from build123d import *

# Parameters (mm, degrees)
SKETCH1_W               = 24.5
SKETCH1_H               = 34.22
BOSS_EXTRUDE1_DEPTH     = 7.5
SKETCH2_W               = 24.5
SKETCH2_H               = 34.22
CUT_EXTRUDE1_DEPTH      = 2.86
SKETCH3_W               = 13.25
SKETCH3_H               = 14.15
CUT_EXTRUDE2_DEPTH      = 3.2
BOSS_EXTRUDE2_START     = -18.25
BOSS_EXTRUDE2_DEPTH     = 36.5
BOSS_EXTRUDE2_START_2   = 7.5
BOSS_EXTRUDE2_2_DEPTH   = 4.5
CUT_EXTRUDE3_DEPTH      = 28.465218004
CUT_EXTRUDE3_DEPTH_BACK = 28.465218004
SKETCH4_R               = 7.25
FILLET1_R               = 6
SKETCH6_R               = 1.475
CUT_EXTRUDE4_DEPTH      = 3


with BuildPart() as part:
    # Sketch1 → Boss-Extrude1 (new body)
    with BuildSketch(Plane.XY):
        Polygon((-12.25, -17.11), (-12.25, 17.11), (12.25, 17.11), (12.25, -17.11), (18.25, -17.11), (14.75, 19.61), (-14.75, 19.61), (-18.25, -17.11), align=None)
        Rectangle(SKETCH1_W, SKETCH1_H)
    extrude(amount=BOSS_EXTRUDE1_DEPTH)

    # Sketch2 → Cut-Extrude1 (cut)
    with BuildSketch(Plane(origin=(0, 0, 0), x_dir=(-1, 0, 0), z_dir=(0, 0, -1))):
        Rectangle(SKETCH2_W, SKETCH2_H)
    extrude(amount=-CUT_EXTRUDE1_DEPTH, mode=Mode.SUBTRACT)

    # Sketch3 → Cut-Extrude2 (cut)
    with BuildSketch(Plane(origin=(0, 0, 2.86), x_dir=(-1, 0, 0), z_dir=(0, 0, -1))):
        with BuildLine():
            Line((-6.625, 6.22), (-6.625, 10.62))
            Line((-6.625, 10.62), (-9.525, 10.62))
            ThreePointArc((-9.525, 10.62), (-11.725, 8.42), (-9.525, 6.22))
            Line((-9.525, 6.22), (-6.625, 6.22))
        make_face()
        with Locations((0, 8.42)):
            Rectangle(SKETCH3_W, SKETCH3_H)
        with BuildLine():
            Line((9.525, 10.62), (6.625, 10.62))
            Line((6.625, 10.62), (6.625, 6.22))
            Line((6.625, 6.22), (9.525, 6.22))
            ThreePointArc((9.525, 6.22), (11.725, 8.42), (9.525, 10.62))
        make_face()
    extrude(amount=-CUT_EXTRUDE2_DEPTH, mode=Mode.SUBTRACT)

    # Boss-Extrude2: read off the stored shape, not the designer's step
    # Boss-Extrude2 outline → Boss-Extrude2 (add)
    with BuildSketch(Plane.YZ.offset(BOSS_EXTRUDE2_START)):
        Polygon((-17.11, 11.359427519), (-17.11, 7.5), (19.61, 7.5), align=None)
    extrude(amount=BOSS_EXTRUDE2_DEPTH)

    # Boss-Extrude2 2 outline → Boss-Extrude2 2 (cut)
    with BuildSketch(Plane.XY.offset(BOSS_EXTRUDE2_START_2)):
        Polygon((14.75, 19.61), (18.25, -17.11), (18.25, 21), (14.617510893, 21), align=None)
        Polygon((-14.75, 19.61), (-14.617510893, 21), (-18.25, 21), (-18.25, -17.11), align=None)
    extrude(amount=BOSS_EXTRUDE2_2_DEPTH, mode=Mode.SUBTRACT)

    # Sketch4 → Cut-Extrude3 (cut, two sides: drawn at the far end of the back side and taken through both)
    with BuildSketch(Plane(origin=(0, 0, 6.06), x_dir=(-1, 0, 0), z_dir=(0, 0, -1)).offset(-CUT_EXTRUDE3_DEPTH_BACK)):
        with Locations(Location((0, 8.42, 0), (0, 0, 17.6648328))):
            Circle(SKETCH4_R)
    extrude(amount=CUT_EXTRUDE3_DEPTH + CUT_EXTRUDE3_DEPTH_BACK, mode=Mode.SUBTRACT)

    # Fillet1
    fillet1_edges = [part.edges().sort_by_distance(p)[0] for p in [
        (-14.75, 19.61, 3.75),
        (14.75, 19.61, 3.75),
    ]]
    fillet(fillet1_edges, radius=FILLET1_R)

    # Sketch6 → Cut-Extrude4 (cut)
    with BuildSketch(Plane(origin=(0, 0, 2.86), x_dir=(-1, 0, 0), z_dir=(0, 0, -1))):
        with Locations((-10.2, 14.86)):
            Circle(SKETCH6_R)
        with Locations(Location((10.2, 14.86, 0), (0, 0, 180))):
            Circle(SKETCH6_R)
    extrude(amount=-CUT_EXTRUDE4_DEPTH, mode=Mode.SUBTRACT)


solid = part.part
Read the model definition and answer for the solid it produces. Units are mm, in the model's axes. A direction names the side the tool comes from. Give positions to 0.01 mm unless a question says otherwise; leave off trailing zeros. Loops run counter-clockwise (first coordinate to the right, second up) from the corner with the lowest first, then second, coordinate; pieces in that order, holes last. Notation, with made-up numbers: M 52.5,19 L 57.5,19 A14 ccw 57.5,27 Z; hole C -23,-27 d5. An arc over 180 degrees is marked long. Write each question's results on one line, items separated by ' | '.
1. A tool of negligible diameter and unlimited length cuts with its end or side. For faces 4 (the face through (-4, 15.495, 4)), 5 (the face through (0, 17.11, 1)), 6 (the face through (-0.26, -2.57, 9.83)), from which of +Z, -Z, +X, -X, +Y, -Y can it reach the whole face along a straight path? Write none if from no direction.
Values:
face 4: -Z | face 5: -Z, -Y | face 6: +Z, +X, -X, +Y
2. Section A-A on y = 8.42 is taken. Give the vertices of the cut face in (x, z) (3 decimals), plus the area to 3 significant figures.
Values:
outline: M -15.817,0 L -12.25,0 L -12.25,2.86 L -11.725,2.86 L -11.725,6.06 L -7.25,6.06 L -7.25,8.676 L -15.817,8.676 Z; M 7.25,6.06 L 11.725,6.06 L 11.725,2.86 L 12.25,2.86 L 12.25,0 L 15.817,0 L 15.817,8.676 L 7.25,8.676 Z | area: 91.4 mm^2
3. Section C-C on x = -10.5 is taken. Give the vertices of the cut face in (y, z).
Values:
outline: M -17.11,2.86 L 6.45,2.86 L 6.45,6.06 L 10.39,6.06 L 10.39,2.86 L 13.42,2.86 L 13.42,5.86 L 16.3,5.86 L 16.3,2.86 L 17.11,2.86 L 17.11,0 L 19.49,0 L 19.49,7.51 L -17.11,11.36 Z
4. Given pin 1 (4.5 mm diameter, centred on x = 3, y = 4, fed in from -Z); pin 2 (1.6 mm diameter, centred on y = 4, z = 4, fed in from -X); pin 3 (4 mm diameter, centred on y = -7.5, z = 4.5, fed in from +X); pin 4 (1.2 mm diameter, centred on x = -4, y = 13, fed in from -Z), each flat-ended and moving along its own axis, determine where each tip first touches the part or whether it passes through.
Values:
pin 1: stops at z = 6.06 | pin 2: stops at x = -16.31 | pin 3: stops at x = 17.52 | pin 4: passes through
5. Section B-B on x = 2.5 is taken. Give the vertices of the cut face in (y, z) (3 decimals).
Values:
outline: M -17.11,2.86 L 1.345,2.86 L 1.345,6.06 L 1.615,6.06 L 1.615,9.391 L -17.11,11.359 Z; M 15.225,6.06 L 15.495,6.06 L 15.495,2.86 L 17.11,2.86 L 17.11,0 L 19.61,0 L 19.61,7.5 L 15.225,7.961 Z
6. Section D-D on y = 14.86 is taken. Give the vertices of the cut face in (x, z) (3 decimals).
Values:
outline: M -15.163,0 L -12.25,0 L -12.25,2.86 L -11.675,2.86 L -11.675,5.86 L -8.725,5.86 L -8.725,2.86 L -6.625,2.86 L -6.625,6.06 L -3.33,6.06 L -3.33,7.999 L -15.163,7.999 Z; M 3.33,6.06 L 6.625,6.06 L 6.625,2.86 L 8.725,2.86 L 8.725,5.86 L 11.675,5.86 L 11.675,2.86 L 12.25,2.86 L 12.25,0 L 15.163,0 L 15.163,7.999 L 3.33,7.999 Z
7. The mould has two halves that part along X. Classify faces 1 (the face through (8, 10.62, 4)), 2 (the face through (0, -17.11, 7)), 3 (the face through (6.625, 13, 4)): pulls with the +X half, pulls with the -X half, needs draft (parallel to the pull), parting line crosses it, or undercut.
Values:
face 1: undercut | face 2: needs draft | face 3: undercut
8. Straight lines are drawn through the part: line 1 (Y direction, x = 0, z = 6); line 2 (Y direction, x = -8.5, z = 4.5); line 3 (Y direction, x = -10.2, z = 3.7) (3 decimals). For each, find the intervals that lie inside material, in ascending order. Write a range as [from, to].
Values:
line 1: y = [-17.11, 1.17], [15.67, 19.61] | line 2: y = [-17.11, 6.22], [10.62, 19.61] | line 3: y = [-17.11, 6.326], [10.514, 13.385], [16.335, 19.541]
